```python
from build123d import *

# Parameters (mm, degrees)
F0_R     = 62.5
F0_R_2   = 58.65
F1_DEPTH = 2
F2_DEPTH = 5


with BuildPart() as f1:
    # F0 (on Top) → F1 (new body)
    with BuildSketch(Plane.XY):
        Circle(F0_R)
        Circle(F0_R_2, mode=Mode.SUBTRACT)
        Circle(F0_R_2)
        with BuildLine():
            Line((-3.191882, -47.253954), (-3.191882, -51.070154))
            Line((-3.191882, -51.070154), (-9.78976, -51.070154))
            ThreePointArc((-9.78976, -51.070154), (-15.862066, -49.52166), (-21.704005, -47.253954))
            Line((-21.704005, -47.253954), (-3.191882, -47.253954))
        make_face(mode=Mode.SUBTRACT)
        with BuildLine():
            Line((-32.918372, -40.253954), (-3.191882, -40.253954))
            Line((-3.191882, -40.253954), (-3.191882, -44.070154))
            Line((-3.191882, -44.070154), (-27.601115, -44.070154))
            ThreePointArc((-27.601115, -44.070154), (-30.319844, -42.245794), (-32.918372, -40.253954))
        make_face(mode=Mode.SUBTRACT)
        with BuildLine():
            Line((-39.977175, -33.253954), (-3.191882, -33.253954))
            Line((-3.191882, -33.253954), (-3.191882, -37.070154))
            Line((-3.191882, -37.070154), (-36.466474, -37.070154))
            ThreePointArc((-36.466474, -37.070154), (-38.269423, -35.205842), (-39.977175, -33.253954))
        make_face(mode=Mode.SUBTRACT)
        with BuildLine():
            Line((-44.885743, -26.253954), (-3.191882, -26.253954))
            Line((-3.191882, -26.253954), (-3.191882, -30.070154))
            Line((-3.191882, -30.070154), (-42.423883, -30.070154))
            ThreePointArc((-42.423883, -30.070154), (-43.696493, -28.188942), (-44.885743, -26.253954))
        make_face(mode=Mode.SUBTRACT)
        with BuildLine():
            Line((-48.304091, -19.253954), (-3.191882, -19.253954))
            Line((-3.191882, -19.253954), (-3.191882, -23.070154))
            Line((-3.191882, -23.070154), (-46.602232, -23.070154))
            ThreePointArc((-46.602232, -23.070154), (-47.491509, -21.179155), (-48.304091, -19.253954))
        make_face(mode=Mode.SUBTRACT)
        with BuildLine():
            Line((-50.535538, -12.253954), (-3.191882, -12.253954))
            Line((-3.191882, -12.253954), (-3.191882, -16.070154))
            Line((-3.191882, -16.070154), (-49.454526, -16.070154))
            ThreePointArc((-49.454526, -16.070154), (-50.031431, -14.172365), (-50.535538, -12.253954))
        make_face(mode=Mode.SUBTRACT)
        with BuildLine():
            Line((-51.733896, -5.253954), (-3.191882, -5.253954))
            Line((-3.191882, -5.253954), (-3.191882, -9.070154))
            Line((-3.191882, -9.070154), (-51.202855, -9.070154))
            ThreePointArc((-51.202855, -9.070154), (-51.503733, -7.166974), (-51.733896, -5.253954))
        make_face(mode=Mode.SUBTRACT)
        with BuildLine():
            Line((-51.970678, 1.746046), (-3.191882, 1.746046))
            Line((-3.191882, 1.746046), (-3.191882, -2.070154))
            Line((-3.191882, -2.070154), (-51.958777, -2.070154))
            ThreePointArc((-51.958777, -2.070154), (-51.999747, -0.162163), (-51.970678, 1.746046))
        make_face(mode=Mode.SUBTRACT)
        with BuildLine():
            Line((7.873907, -51.400405), (2.896511, -49.572833))
            Line((2.896511, -49.572833), (2.896511, -45.902099))
            Line((2.896511, -45.902099), (14.289776, -49.998023))
            ThreePointArc((14.289776, -49.998023), (11.104003, -50.800602), (7.873907, -51.400405))
        make_face(mode=Mode.SUBTRACT)
        with BuildLine():
            Line((19.31125, -48.281214), (2.896511, -41.941576))
            Line((2.896511, -41.941576), (2.896511, -38.46404))
            Line((2.896511, -38.46404), (23.862975, -46.201281))
            ThreePointArc((23.862975, -46.201281), (21.612149, -47.296036), (19.31125, -48.281214))
        make_face(mode=Mode.SUBTRACT)
        with BuildLine():
            Line((27.758943, -43.970912), (2.896511, -34.795944))
            Line((2.896511, -34.795944), (2.896511, -30.815715))
            Line((2.896511, -30.815715), (31.400508, -41.448861))
            ThreePointArc((31.400508, -41.448861), (29.606593, -42.74868), (27.758943, -43.970912))
        make_face(mode=Mode.SUBTRACT)
        with BuildLine():
            ThreePointArc((37.372623, -36.156424), (36.007063, -37.516548), (34.592037, -38.825133))
            Line((34.592037, -38.825133), (2.896511, -27.206514))
            Line((2.896511, -27.206514), (2.896511, -23.518527))
            Line((2.896511, -23.518527), (37.372623, -36.156424))
        make_face(mode=Mode.SUBTRACT)
        with BuildLine():
            Line((39.978156, -33.252775), (2.896511, -19.830042))
            Line((2.896511, -19.830042), (2.896511, -16.004948))
            Line((2.896511, -16.004948), (42.286384, -30.263208))
            ThreePointArc((42.286384, -30.263208), (41.159422, -31.778955), (39.978156, -33.252775))
        make_face(mode=Mode.SUBTRACT)
        with BuildLine():
            Line((44.263286, -27.290319), (2.896511, -12.316464))
            Line((2.896511, -12.316464), (2.896511, -8.503364))
            Line((2.896511, -8.503364), (46.063064, -24.128698))
            ThreePointArc((46.063064, -24.128698), (45.190833, -25.725253), (44.263286, -27.290319))
        make_face(mode=Mode.SUBTRACT)
        with BuildLine():
            Line((2.896511, -4.746575), (2.896511, -3.21917))
            Line((2.896511, -3.21917), (8.751221, -3.21917))
            Line((8.751221, -3.21917), (48.754682, -18.082614))
            ThreePointArc((48.754682, -18.082614), (48.166824, -19.594823), (47.532074, -21.087957))
            Line((47.532074, -21.087957), (2.896511, -4.746575))
        make_face(mode=Mode.SUBTRACT)
        with BuildLine():
            Line((49.812785, -14.922684), (18.313957, -3.21917))
            Line((18.313957, -3.21917), (29.242799, -3.21917))
            Line((29.242799, -3.21917), (50.799583, -11.10866))
            ThreePointArc((50.799583, -11.10866), (50.342317, -13.025021), (49.812785, -14.922684))
        make_face(mode=Mode.SUBTRACT)
        with BuildLine():
            Line((51.415095, -7.777406), (39.14706, -3.21917))
            Line((39.14706, -3.21917), (49.597766, -3.21917))
            Line((49.597766, -3.21917), (51.828544, -4.219248))
            ThreePointArc((51.828544, -4.219248), (51.652467, -6.001889), (51.415095, -7.777406))
        make_face(mode=Mode.SUBTRACT)
        with BuildLine():
            Line((-51.259211, 8.746046), (-3.191882, 8.746046))
            Line((-3.191882, 8.746046), (-3.191882, 4.929846))
            Line((-3.191882, 4.929846), (-51.765786, 4.929846))
            ThreePointArc((-51.765786, 4.929846), (-51.547826, 6.842636), (-51.259211, 8.746046))
        make_face(mode=Mode.SUBTRACT)
        with BuildLine():
            Line((-49.558673, 15.746046), (-3.191882, 15.746046))
            Line((-3.191882, 15.746046), (-3.191882, 11.929846))
            Line((-3.191882, 11.929846), (-50.61303, 11.929846))
            ThreePointArc((-50.61303, 11.929846), (-50.122184, 13.847984), (-49.558673, 15.746046))
        make_face(mode=Mode.SUBTRACT)
        with BuildLine():
            Line((-46.761281, 22.746046), (-3.191882, 22.746046))
            Line((-3.191882, 22.746046), (-3.191882, 18.929846))
            Line((-3.191882, 18.929846), (-48.432024, 18.929846))
            ThreePointArc((-48.432024, 18.929846), (-47.634884, 20.854684), (-46.761281, 22.746046))
        make_face(mode=Mode.SUBTRACT)
        with BuildLine():
            Line((-42.651761, 29.746046), (-3.191882, 29.746046))
            Line((-3.191882, 29.746046), (-3.191882, 25.929846))
            Line((-3.191882, 25.929846), (-45.073751, 25.929846))
            ThreePointArc((-45.073751, 25.929846), (-43.904239, 27.864274), (-42.651761, 29.746046))
        make_face(mode=Mode.SUBTRACT)
        with BuildLine():
            Line((-36.793044, 36.746046), (-3.191882, 36.746046))
            Line((-3.191882, 36.746046), (-3.191882, 32.929846))
            Line((-3.191882, 32.929846), (-40.244568, 32.929846))
            ThreePointArc((-40.244568, 32.929846), (-38.566038, 34.880664), (-36.793044, 36.746046))
        make_face(mode=Mode.SUBTRACT)
        with BuildLine():
            Line((-28.111981, 43.746046), (-3.191882, 43.746046))
            Line((-3.191882, 43.746046), (-3.191882, 39.929846))
            Line((-3.191882, 39.929846), (-33.31077, 39.929846))
            ThreePointArc((-33.31077, 39.929846), (-30.770593, 41.918619), (-28.111981, 43.746046))
        make_face(mode=Mode.SUBTRACT)
        with BuildLine():
            ThreePointArc((-22.396194, 46.929846), (-16.981001, 49.149218), (-11.350719, 50.746046))
            Line((-11.350719, 50.746046), (-3.191882, 50.746046))
            Line((-3.191882, 50.746046), (-3.191882, 46.929846))
            Line((-3.191882, 46.929846), (-22.396194, 46.929846))
        make_face(mode=Mode.SUBTRACT)
        with BuildLine():
            Line((8.782855, 2.79247), (2.896511, 2.79247))
            Line((2.896511, 2.79247), (2.896511, 4.687412))
            Line((2.896511, 4.687412), (47.540674, 21.068563))
            ThreePointArc((47.540674, 21.068563), (48.236133, 19.423579), (48.874694, 17.755684))
            Line((48.874694, 17.755684), (8.782855, 2.79247))
        make_face(mode=Mode.SUBTRACT)
        with BuildLine():
            Line((46.099099, 24.059782), (2.896511, 8.247841))
            Line((2.896511, 8.247841), (2.896511, 12.165699))
            Line((2.896511, 12.165699), (44.300966, 27.22911))
            ThreePointArc((44.300966, 27.22911), (45.227802, 25.660202), (46.099099, 24.059782))
        make_face(mode=Mode.SUBTRACT)
        with BuildLine():
            Line((42.353825, 30.16875), (2.896511, 15.764672))
            Line((2.896511, 15.764672), (2.896511, 19.787056))
            Line((2.896511, 19.787056), (40.094616, 33.11226))
            ThreePointArc((40.094616, 33.11226), (41.250484, 31.660663), (42.353825, 30.16875))
        make_face(mode=Mode.SUBTRACT)
        with BuildLine():
            Line((37.661768, 35.855142), (2.896511, 23.033189))
            Line((2.896511, 23.033189), (2.896511, 27.158916))
            Line((2.896511, 27.158916), (34.637542, 38.784542))
            ThreePointArc((34.637542, 38.784542), (36.179316, 37.350463), (37.661768, 35.855142))
        make_face(mode=Mode.SUBTRACT)
        with BuildLine():
            ThreePointArc((51.467824, 7.420449), (51.695994, 5.614641), (51.860825, 3.801954))
            Line((51.860825, 3.801954), (49.609106, 2.79247))
            Line((49.609106, 2.79247), (39.046496, 2.79247))
            Line((39.046496, 2.79247), (51.467824, 7.420449))
        make_face(mode=Mode.SUBTRACT)
        with BuildLine():
            Line((50.851188, 10.869989), (29.255319, 2.79247))
            Line((29.255319, 2.79247), (18.217992, 2.79247))
            Line((18.217992, 2.79247), (49.896269, 14.64112))
            ThreePointArc((49.896269, 14.64112), (50.409006, 12.764487), (50.851188, 10.869989))
        make_face(mode=Mode.SUBTRACT)
        with BuildLine():
            Line((24.35126, 45.945796), (2.896511, 38.12946))
            Line((2.896511, 38.12946), (2.896511, 41.930046))
            Line((2.896511, 41.930046), (19.827624, 48.071461))
            ThreePointArc((19.827624, 48.071461), (22.114996, 47.06301), (24.35126, 45.945796))
        make_face(mode=Mode.SUBTRACT)
        with BuildLine():
            Line((31.694718, 41.224324), (2.896511, 30.533878))
            Line((2.896511, 30.533878), (2.896511, 34.331668))
            Line((2.896511, 34.331668), (28.38323, 43.570543))
            ThreePointArc((28.38323, 43.570543), (30.061872, 42.429752), (31.694718, 41.224324))
        make_face(mode=Mode.SUBTRACT)
        with BuildLine():
            Line((14.515265, 49.933026), (2.896511, 45.727838))
            Line((2.896511, 45.727838), (2.896511, 49.406949))
            Line((2.896511, 49.406949), (8.121136, 51.361923))
            ThreePointArc((8.121136, 51.361923), (11.340727, 50.74828), (14.515265, 49.933026))
        make_face(mode=Mode.SUBTRACT)
    extrude(amount=-F1_DEPTH)

    # F0 (on Top) → F2 (join)
    with BuildSketch(Plane.XY):
        Circle(F0_R)
        Circle(F0_R_2, mode=Mode.SUBTRACT)
    extrude(amount=F2_DEPTH)


solid = f1.part
```
The listing builds one solid part. Answer for the finished solid, in the listing's coordinates (mm). A direction names the side the tool comes from. Coordinates: 2 decimals unless noted, no trailing zeros. Write each loop counter-clockwise with the first axis right and the second up, starting at its lowest first coordinate (ties: lowest second). Pieces come first, ordered by that corner, then holes. Notation, with made-up numbers: (42, -13) - (93, -13) arc R33 cw to (93, 22) - close; hole circle Ø2 at (32, -27.75). An arc over 180 degrees is marked (long way). Return JSON: item names as keys, results as strings. Group by question number.
1. Which of the six approach directions +Z, -Z, +X, -X, +Y, -Y give full straight-line access (tool end or side, diameter ignored) to faces 1 (the cylindrical face through (-43.227, 39.638, 2.465)), 2 (the flat face through (11.219, -45.156, -0.986))?
2. A cutting plane is placed at B-B, the plane x = 0. Determine the outline of the cut face in (y, z).
3. A cutting plane is placed at C-C, the plane z = 1.5. Determine the outline of the cut face in (x, y), plus the area to 3 significant figures.
4. A cutting plane is placed at D-D, the plane x = -13.5. Give the number of separate pieces and of enclosed holes in the cut face, plus the area to 3 significant figures.
5. A cutting plane is placed at A-A, the plane y = 0. Determine the outline of the cut face in (x, z).
6. Straight lines are drawn through the part: L1, parallel to Y at x = 0, z = 3.1; L2, parallel to Y at x = 30.5, z = 3.25; L3, parallel to Z at x = -56.5, y = 3.5. For each, find the intervals that lie inside material, in ascending order.
7. Given pin 1 (1 mm diameter, centred on y = -42.5, z = -1, fed in from -X); pin 2 (0.6 mm diameter, centred on x = 5.5, z = -1, fed in from +Y); pin 3 (3 mm diameter, centred on y = -36, z = 4, fed in from +X), each flat-ended and moving along its own axis, determine where each tip first touches the part or whether it passes through.
Ans:
{
 "1": {"face 1": "+Z", "face 2": "+Z, -Z"},
 "2": {"outline": "(-62.5, -2) - (62.5, -2) - (62.5, 5) - (58.65, 5) - (58.65, 0) - (-58.65, 0) - (-58.65, 5) - (-62.5, 5) - close"},
 "3": {"outline": "circle Ø125 at (0, 0); hole circle Ø117.3 at (0, 0)", "area": "1,470 mm²"},
 "4": {"separate pieces": "16", "enclosed holes": "0", "area": "172 mm²"},
 "5": {"outline": "(-62.5, -2) - (-52, -2) - (-52, 0) - (-58.65, 0) - (-58.65, 5) - (-62.5, 5) - close; (-3.19, -2) - (62.5, -2) - (62.5, 5) - (58.65, 5) - (58.65, 0) - (-3.19, 0) - close"},
 "6": {"L1": "-62.5 to -58.65, 58.65 to 62.5", "L2": "-54.55 to -50.1, 50.1 to 54.55", "L3": "-2 to 0"},
 "7": {"pin 1": "x = -46.28", "pin 2": "y = 62.28", "pin 3": "x = 52.12"}
}
